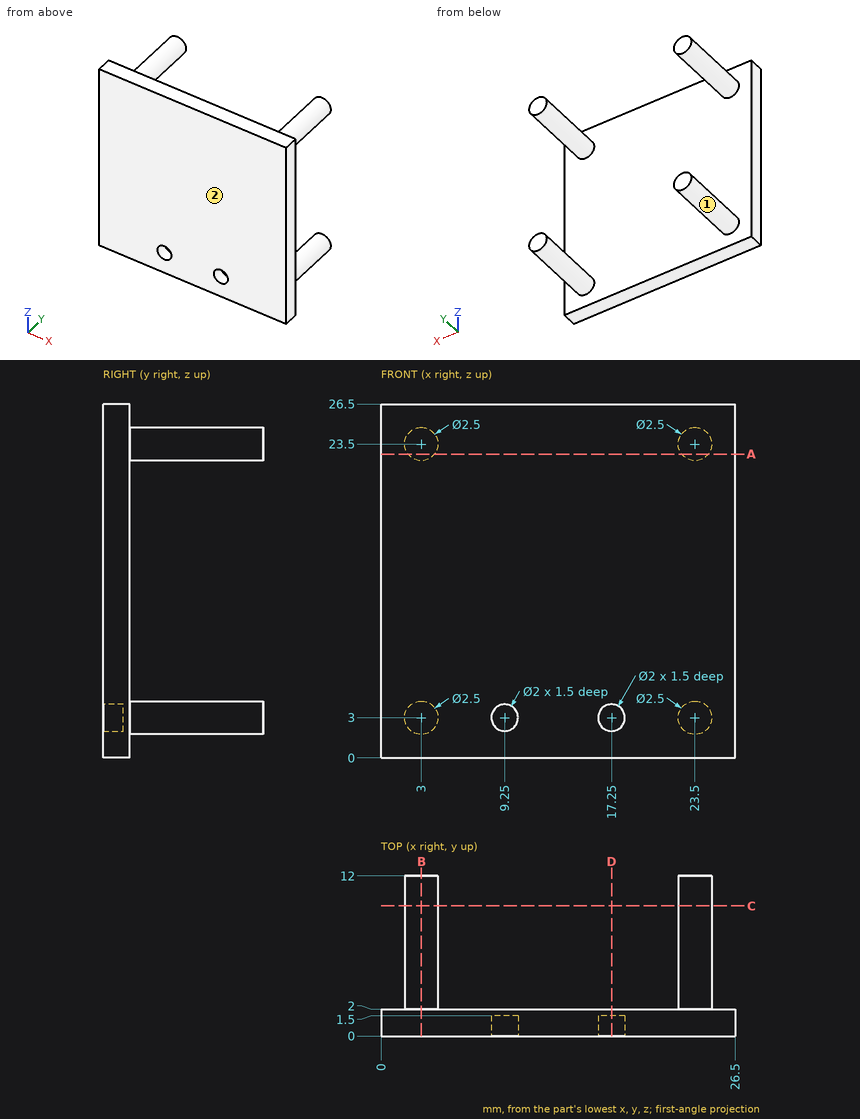
Drawing for the job (mm, zero at the part's lowest x, y, z). Round coordinates to 2 decimals unless told otherwise and drop trailing zeros. Write each loop counter-clockwise with the first axis right and the second up, starting at its lowest first coordinate (ties: lowest second). Pieces come first, ordered by that corner, then holes. Notation, with made-up numbers: (-10, -37) - (26, -37) arc R13 ccw to (26, -30) - close; hole circle Ø6 at (-32.75, -3). An arc over 180 degrees is marked (long way). Use CSV: the item, a comma, the result in double quotes.
(1) Wall check: line 1 (X direction, y = 1.15, z = 3); line 2 (X direction, y = 2.75, z = 23.25); line 3 (Y direction, x = 3.75, z = 25.25). Give the ranges that are in metal, low to high.
Response:
line 1,"0 to 8.25, 10.25 to 16.25, 18.25 to 26.5"
line 2,"1.78 to 4.22, 22.28 to 24.72"
line 3,"0 to 2"
(2) Band-saw the part on B-B (x = 3). Write the cut outline in (y, z), plus the area to 3 significant figures.
Response:
outline,"(0, 0) - (2, 0) - (2, 1.75) - (12, 1.75) - (12, 4.25) - (2, 4.25) - (2, 22.25) - (12, 22.25) - (12, 24.75) - (2, 24.75) - (2, 26.5) - (0, 26.5) - close"
area,"103 mm²"
(3) Pin check, flat tips, straight feed: P1, Ø1.5, axis at y = 9, z = 23.5, coming from the +X side; P2, Ø4, axis at x = 15, z = 23.5, coming from the +Y side; P3, Ø1.8, axis at x = 17.25, z = 3, coming from the -Y side. Stop position of each tip, or through.
Response:
P1,"x = 24.75"
P2,"y = 2"
P3,"y = 1.5"
(4) Band-saw the part on D-D (x = 17.25). Write the cut outline in (y, z), plus the area to 3 significant figures.
Response:
outline,"(0, 0) - (2, 0) - (2, 26.5) - (0, 26.5) - (0, 4) - (1.5, 4) - (1.5, 2) - (0, 2) - close"
area,"50.0 mm²"
(5) Mould opens along Z. For the marked faces 1 and 2 say: pulls with the +Z half, pulls with the -Z half, needs draft (parallel to the pull), parting line crosses it, or undercut.
Response:
face 1,"undercut"
face 2,"needs draft"
(6) Band-saw the part on C-C (y = 9.75). Write the cut outline in (x, z).
Response:
outline,"circle Ø2.5 at (3, 3); circle Ø2.5 at (3, 23.5); circle Ø2.5 at (23.5, 3); circle Ø2.5 at (23.5, 23.5)"
(7) Band-saw the part on A-A (z = 22.75). Write the cut outline in (x, y), plus the area to 3 significant figures.
Response:
outline,"(0, 0) - (26.5, 0) - (26.5, 2) - (24.5, 2) - (24.5, 12) - (22.5, 12) - (22.5, 2) - (4, 2) - (4, 12) - (2, 12) - (2, 2) - (0, 2) - close"
area,"93.0 mm²"
